```python
from build123d import *

# Parameters (mm, degrees)
EXTRUSION1_DEPTH        = 22.64
ENL_V_MAT_EXTRU_1_DEPTH = 24.262299972
ESQUISSE3_R             = 0.4
ENL_V_MAT_EXTRU_2_DEPTH = 2.5
ESQUISSE5_R             = 0.25
EXTRUSION2_DEPTH        = 3


with BuildPart() as part:
    # Esquisse1 → Extrusion1 (new body)
    with BuildSketch(Plane(origin=(0, 0, 0), x_dir=(0, 0, -1), z_dir=(1, 0, 0))):
        Polygon((-2.25, 1.75), (-2.25, 3), (-5.05, 3), (-5.05, 0), (5.05, 0), (5.05, 3), (2.25, 3), (2.25, 1.75), align=None)
    extrude(amount=EXTRUSION1_DEPTH)

    # Esquisse2 → Enlèv. mat.-Extru.1 (cut, through all)
    with BuildSketch(Plane(origin=(0, 1.75, 0), x_dir=(-1, 0, 0), z_dir=(0, 1, 0))):
        with BuildLine():
            Line((0, -1), (0, 1))
            ThreePointArc((0, 1), (-1, 0), (0, -1))
        make_face()
    extrude(amount=-ENL_V_MAT_EXTRU_1_DEPTH, mode=Mode.SUBTRACT)

    # Esquisse3 → Enlèv. mat.-Extru.2 (cut)
    with BuildSketch(Plane(origin=(0, 3, 0), x_dir=(-1, 0, 0), z_dir=(0, 1, 0))):
        with Locations(Location((-1.16, 3.65, 0), (0, 0, 90))):
            Circle(ESQUISSE3_R)
        with Locations(Location((-1.16, -3.65, 0), (0, 0, 270))):
            Circle(ESQUISSE3_R)
        with Locations(Location((-3.7, 3.65, 0), (0, 0, 90))):
            Circle(ESQUISSE3_R)
        with Locations(Location((-3.7, -3.65, 0), (0, 0, 270))):
            Circle(ESQUISSE3_R)
        with Locations(Location((-6.24, 3.65, 0), (0, 0, 90))):
            Circle(ESQUISSE3_R)
        with Locations(Location((-6.24, -3.65, 0), (0, 0, 270))):
            Circle(ESQUISSE3_R)
        with Locations(Location((-8.78, 3.65, 0), (0, 0, 90))):
            Circle(ESQUISSE3_R)
        with Locations(Location((-8.78, -3.65, 0), (0, 0, 270))):
            Circle(ESQUISSE3_R)
        with Locations(Location((-11.32, 3.65, 0), (0, 0, 90))):
            Circle(ESQUISSE3_R)
        with Locations(Location((-11.32, -3.65, 0), (0, 0, 270))):
            Circle(ESQUISSE3_R)
        with Locations(Location((-13.86, 3.65, 0), (0, 0, 90))):
            Circle(ESQUISSE3_R)
        with Locations(Location((-13.86, -3.65, 0), (0, 0, 270))):
            Circle(ESQUISSE3_R)
        with Locations(Location((-16.4, 3.65, 0), (0, 0, 90))):
            Circle(ESQUISSE3_R)
        with Locations(Location((-16.4, -3.65, 0), (0, 0, 270))):
            Circle(ESQUISSE3_R)
        with Locations(Location((-18.94, 3.65, 0), (0, 0, 90))):
            Circle(ESQUISSE3_R)
        with Locations(Location((-18.94, -3.65, 0), (0, 0, 270))):
            Circle(ESQUISSE3_R)
        with Locations(Location((-21.48, 3.65, 0), (0, 0, 90))):
            Circle(ESQUISSE3_R)
        with Locations(Location((-21.48, -3.65, 0), (0, 0, 270))):
            Circle(ESQUISSE3_R)
    extrude(amount=-ENL_V_MAT_EXTRU_2_DEPTH, mode=Mode.SUBTRACT)

    # Esquisse5 → Extrusion2 (add)
    with BuildSketch(Plane.XZ):
        with Locations(Location((1.16, 3.81, 0), (0, 0, 90))):
            Circle(ESQUISSE5_R)
        with Locations(Location((1.16, -3.81, 0), (0, 0, 90))):
            Circle(ESQUISSE5_R)
        with Locations(Location((3.7, -3.81, 0), (0, 0, 90))):
            Circle(ESQUISSE5_R)
        with Locations(Location((3.7, 3.81, 0), (0, 0, 90))):
            Circle(ESQUISSE5_R)
        with Locations(Location((6.24, -3.81, 0), (0, 0, 90))):
            Circle(ESQUISSE5_R)
        with Locations(Location((6.24, 3.81, 0), (0, 0, 90))):
            Circle(ESQUISSE5_R)
        with Locations(Location((8.78, -3.81, 0), (0, 0, 90))):
            Circle(ESQUISSE5_R)
        with Locations(Location((8.78, 3.81, 0), (0, 0, 90))):
            Circle(ESQUISSE5_R)
        with Locations(Location((11.32, -3.81, 0), (0, 0, 90))):
            Circle(ESQUISSE5_R)
        with Locations(Location((11.32, 3.81, 0), (0, 0, 90))):
            Circle(ESQUISSE5_R)
        with Locations(Location((13.86, -3.81, 0), (0, 0, 90))):
            Circle(ESQUISSE5_R)
        with Locations(Location((13.86, 3.81, 0), (0, 0, 90))):
            Circle(ESQUISSE5_R)
        with Locations(Location((16.4, -3.81, 0), (0, 0, 90))):
            Circle(ESQUISSE5_R)
        with Locations(Location((16.4, 3.81, 0), (0, 0, 90))):
            Circle(ESQUISSE5_R)
        with Locations(Location((18.94, -3.81, 0), (0, 0, 90))):
            Circle(ESQUISSE5_R)
        with Locations(Location((18.94, 3.81, 0), (0, 0, 90))):
            Circle(ESQUISSE5_R)
        with Locations(Location((21.48, -3.81, 0), (0, 0, 90))):
            Circle(ESQUISSE5_R)
        with Locations(Location((21.48, 3.81, 0), (0, 0, 90))):
            Circle(ESQUISSE5_R)
    extrude(amount=EXTRUSION2_DEPTH)


solid = part.part
```
Geometry check sheet. Reference: the model listing, model coordinates, mm. A direction names the side the tool comes from. Round coordinates to 2 decimals unless told otherwise and drop trailing zeros. Order: outer loops, then holes, each group sorted by start corner. A loop starts at its lowest first (then second) coordinate and runs counter-clockwise, first axis right, second up. Notation, with made-up numbers: (79, 86) -> (131, 86) arc R27 ccw to (131, 117) -> close; hole circle Ø11 at (-38.5, -14). An arc over 180 degrees is marked (long way). Return JSON: item names as keys, results as strings. Group by question number.
Q1. Section check B-B, the plane x = 2.25. Record the boundary of the cut face in (y, z).
Q2. Tool access check on faces 5 (the flat face through (0, 2, 4)), 6 (the cylindrical face through (10.965, 1.768, 3.835)), 7 (the flat face through (11, 1.75, 0)). Record the directions out of +Z, -Z, +X, -X, +Y, -Y that give a thin tool (end or side, any length) a straight path to the whole face; none if there is none.
Q3. Gauge pin test, flat end, axial feed: pin 1 (1.5 mm diameter, centred on x = 6, z = -2, fed in from -Y). Record the tip position at first contact, or that the pin passes through.
Q4. Release check for a two-part mould opening along Z. For faces 1 (the flat face through (11, 2, 2.25)), 2 (the cylindrical face through (6.595, 1.768, -3.835)), 3 (the flat face through (11.2, 3, -4.3)), 4 (the flat face through (11, 1, -5.05)) record: released by +Z, released by -Z, zero draft, split by the parting line, or undercut.
Q5. Material ranges on probe 1 along Z at (x, y) = (9, 0.8); probe 2 along Y at (x, z) = (18.25, -0.5); probe 3 along Y at (x, z) = (12.75, 3), recorded low to high. Write a range as from..to.
Q6. Section check A-A, the plane y = 2.15. Count the separate pieces of the cut face and the enclosed holes in it, plus the area to 3 significant figures.
Numbers:
{
 "1": {"outline": "(0, -5.05) -> (3, -5.05) -> (3, -2.25) -> (1.75, -2.25) -> (1.75, 2.25) -> (3, 2.25) -> (3, 5.05) -> (0, 5.05) -> close"},
 "2": {"face 5": "+Z, -Z, -X, +Y, -Y", "face 6": "+Y", "face 7": "+X, -X, +Y"},
 "3": {"pin 1": "y = 0"},
 "4": {"face 1": "undercut", "face 2": "undercut", "face 3": "zero draft", "face 4": "released by -Z"},
 "5": {"probe 1": "-5.05..-3.98, -3.32..3.32, 3.98..5.05", "probe 2": "0..1.75", "probe 3": "0..3"},
 "6": {"separate pieces": "2", "enclosed holes": "18", "area": "118 mm^2"}
}
